Here's the drawing with two shaded views (mm, measured from the low corner). I have some questions. Round coordinates to 2 decimals unless told otherwise and drop trailing zeros. Write each loop counter-clockwise with the first axis right and the second up, starting at its lowest first coordinate (ties: lowest second). Pieces come first, ordered by that corner, then holes. Notation, with made-up numbers: M 86,-15.5 L 122,-15.5 A27 ccw 122,20.5 Z; hole C -33,36 d3. An arc over 180 degrees is marked long. Write item = value, one per line. Start each with the question number.
(1) Will these pins go through, and if not, where does the flat tip stop? pin 1 Ø6 at (x, y) = (33.5, 19.5) entering from -Z; pin 2 Ø2 at (y, z) = (9.5, 19.5) entering from +X; pin 3 Ø4 at (x, y) = (44, 8) entering from -Z.
(2) I want a section at D-D (z = 14). List the corners of the cut face in (x, y) for me.
(3) I need wall thicknesses on line 1 along Y through (x, z) = (24.5, 21.5); line 2 along Y through (x, z) = (42.5, 4.5); line 3 along X through (y, z) = (18.25, 15). Which ranges of each line are inside material? Lowest first, please.
(4) I want a section at C-C (y = 4). List the corners of the cut face in (x, z) for me (3 decimals), and give its area (3 significant figures).
(5) I want a section at A-A (x = 44.5). List the corners of the cut face in (y, z) for me.
(6) I want a section at B-B (y = 17.5). List the corners of the cut face in (x, z) for me.
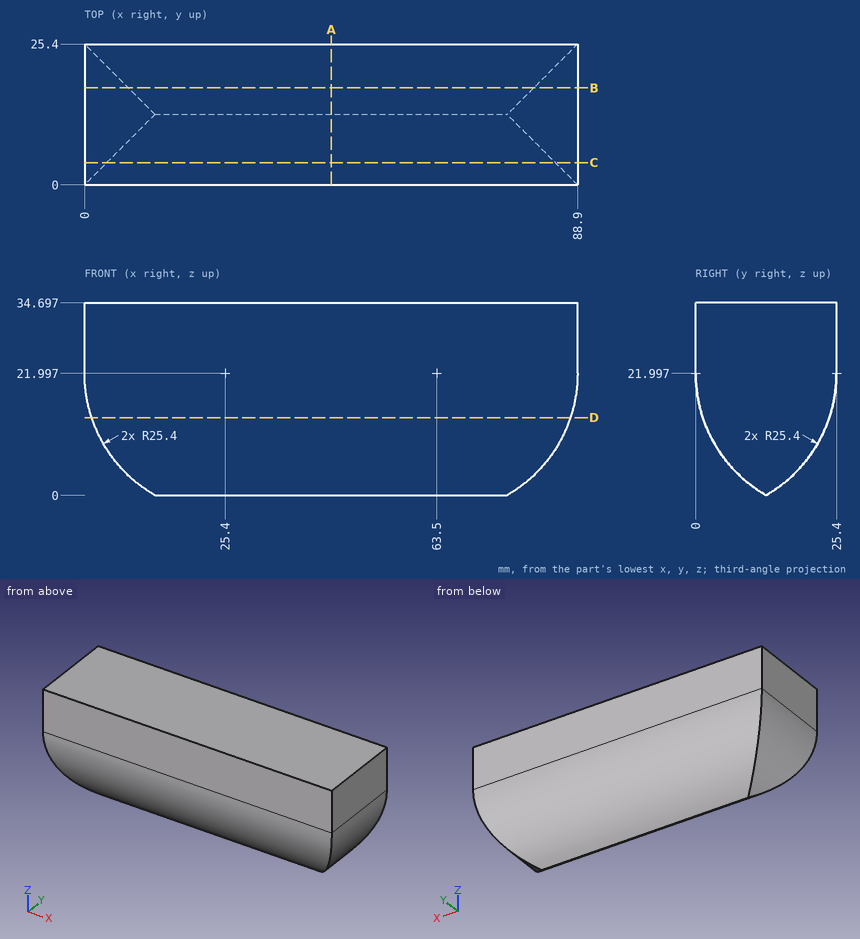
Returned:
q1.pin_1 = 2.69
q1.pin_2 = 88.86
q1.pin_3 = 1.8
q2.outline = M 1.29,1.29 L 87.61,1.29 L 87.61,24.11 L 1.29,24.11 Z
q3.line_1 = 0 to 25.4
q3.line_2 = 6.99 to 18.41
q3.line_3 = 0.98 to 87.92
q4.outline = M 0,21.997 A25.4 ccw 4,8.315 L 84.9,8.315 A25.4 ccw 88.9,21.997 L 88.9,34.697 L 0,34.697 Z
q4.area = 2,310 mm²
q5.outline = M 0,22 A25.4 ccw 12.7,0 A25.4 ccw 25.4,22 L 25.4,34.7 L 0,34.7 Z
q6.outline = M 0,22 A25.4 ccw 7.9,3.59 L 81,3.59 A25.4 ccw 88.9,22 L 88.9,34.7 L 0,34.7 Z
